Can you work these out from the drawing? Everything is in mm from the part's minimum corner. A direction names the side the tool comes from. Round coordinates to 2 decimals unless told otherwise and drop trailing zeros. Write each loop counter-clockwise with the first axis right and the second up, starting at its lowest first coordinate (ties: lowest second). Pieces come first, ordered by that corner, then holes. Notation, with made-up numbers: (-18.75, 37.25) -> (-5.75, 37.25) arc R19 cw to (-5.75, 44.25) -> close; hole circle Ø11 at (-20.75, 0). An arc over 180 degrees is marked (long way). Write item = value, one per line. Start each with the question number.
1) Imagine slicing it at A-A, the plane z = 13.5. Please give me the cut outline in (x, y).
2) Imagine slicing it at D-D, the plane y = 16.5. Please give me the cut outline in (x, z), then the cut area to 3 significant figures.
3) Imagine slicing it at B-B, the plane y = 5. Please give me the cut outline in (x, z).
4) Thinking about a two-plate mould opening in Y: for the marked faces 1, 2 and 3, which applies, +Y half, -Y half, draft (parallel to the pull), parting line (faces both ways), or undercut?
5) For the marked faces 4 and 5, which set-ups out of +Z, -Z, +X, -X, +Y, -Y let a thin tool reach every point of the face, with its end or its side?
6) Imagine slicing it at C-C, the plane x = 5.75. Please give me the cut outline in (y, z).
7) I'm going to push flat-ended pins straight in: pin 1 (3 mm diameter, centred on y = 12.5, z = 10, fed in from +X); pin 2 (5 mm diameter, centred on y = 5, z = 4, fed in from +X); pin 3 (1.5 mm diameter, centred on y = 14, z = 5.5, fed in from +X); pin 4 (4 mm diameter, centred on x = 5, y = 16, fed in from -Z). Where does each tip first touch, or does it pass through?
8) If I drill on line 1 (Z direction, x = 1.3, y = 5); line 2 (Y direction, x = 5, z = 8.75); line 3 (X direction, y = 9, z = 16.5), over which ranges is the centre line in solid material (lowest first)?
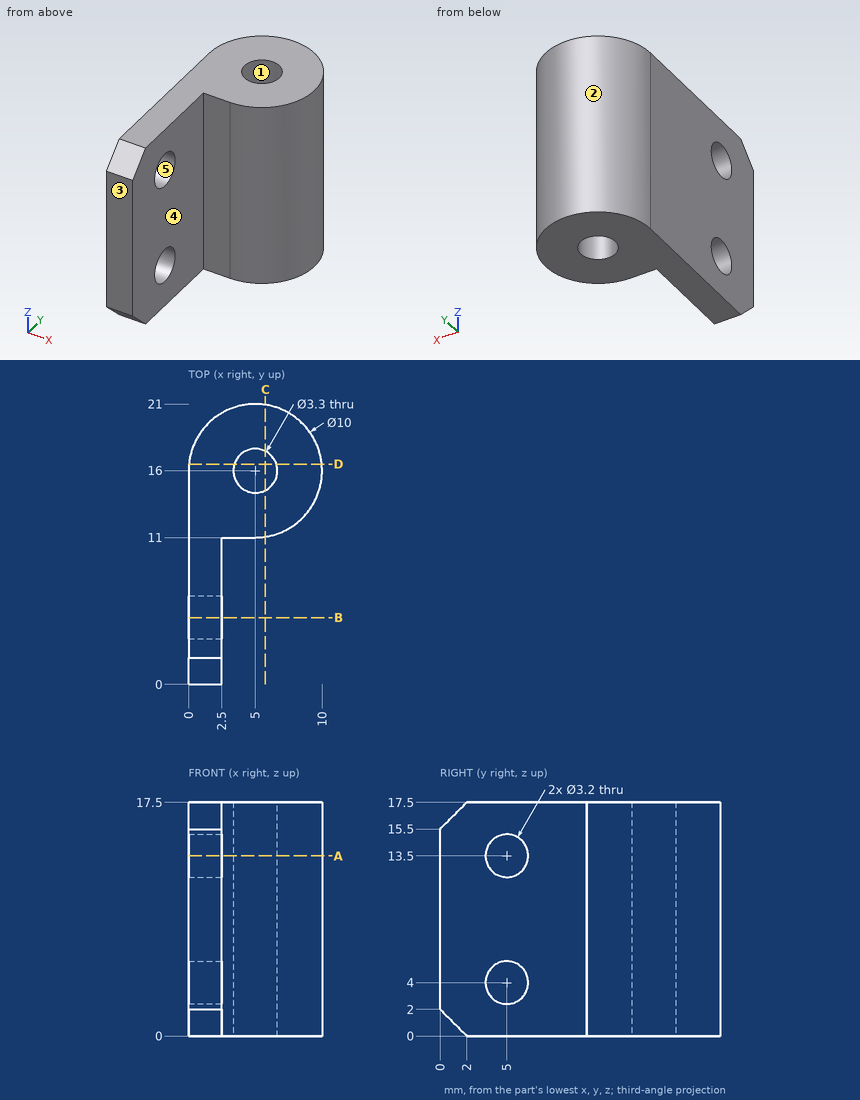
Reported:
q1.outline = (0, 0) -> (2.5, 0) -> (2.5, 3.4) -> (0, 3.4) -> close; (0, 6.6) -> (2.5, 6.6) -> (2.5, 11) -> (5, 11) arc R5 ccw (long way) to (0, 16) -> close; hole circle Ø3.3 at (5, 16)
q2.outline = (0.03, 0) -> (3.43, 0) -> (3.43, 17.5) -> (0.03, 17.5) -> close; (6.57, 0) -> (9.97, 0) -> (9.97, 17.5) -> (6.57, 17.5) -> close
q2.area = 119 mm²
q3.outline = (0, 0) -> (2.5, 0) -> (2.5, 2.4) -> (0, 2.4) -> close; (0, 5.6) -> (2.5, 5.6) -> (2.5, 11.9) -> (0, 11.9) -> close; (0, 15.1) -> (2.5, 15.1) -> (2.5, 17.5) -> (0, 17.5) -> close
q4.face_1 = undercut
q4.face_2 = parting line
q4.face_3 = -Y half
q5.face_4 = +Z, -Z, +X, -Y
q5.face_5 = +X, -X
q6.outline = (11.06, 0) -> (14.53, 0) -> (14.53, 17.5) -> (11.06, 17.5) -> close; (17.47, 0) -> (20.94, 0) -> (20.94, 17.5) -> (17.47, 17.5) -> close
q7.pin_1 = 9.58
q7.pin_2 = 2.5
q7.pin_3 = 9.84
q7.pin_4 = 0
q8.line_1 = 0 to 2.4, 5.6 to 11.9, 15.1 to 17.5
q8.line_2 = 11 to 14.35, 17.65 to 21
q8.line_3 = 0 to 2.5
